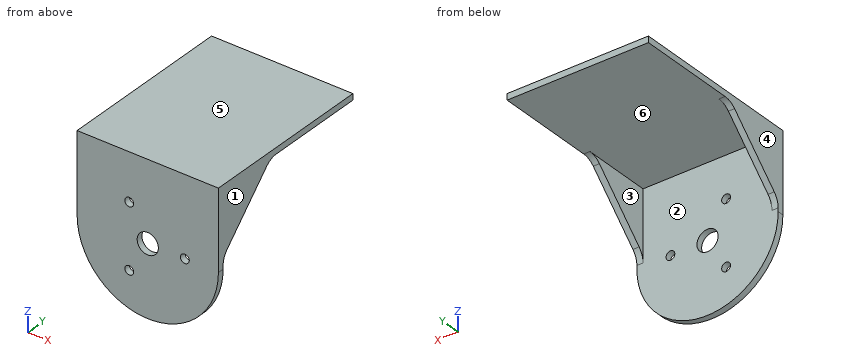
from build123d import *

# Parameters (mm, degrees)
SKETCH1_R            = 2.5
SKETCH1_R_2          = 6
BOSS_EXTRUDE1_DEPTH  = 3.5
SKETCH1_3_W          = 80
SKETCH1_3_H          = 3.5
BOSS_EXTRUDE2_DEPTH  = 100
BOSS_EXTRUDE3_DEPTH  = 3.5
FILLET1_R            = 10
FILLET1_OF_MIRROR1_R = 10


with BuildPart() as part:
    # Sketch1 → Boss-Extrude1 (new body)
    with BuildSketch(Plane(origin=(0, 0, 0), x_dir=(1, 0, 0), z_dir=(0, 1, 0))):
        with BuildLine():
            ThreePointArc((40, 0), (0, 40), (-40, 0))
            Line((-40, 0), (-40, -41.5))
            Line((-40, -41.5), (40, -41.5))
            Line((40, -41.5), (40, 0))
        make_face()
        with Locations((21, 0)):
            Circle(SKETCH1_R, mode=Mode.SUBTRACT)
        with Locations((-10.5, -18.186533479)):
            Circle(SKETCH1_R, mode=Mode.SUBTRACT)
        with Locations((-10.5, 18.186533479)):
            Circle(SKETCH1_R, mode=Mode.SUBTRACT)
        Circle(SKETCH1_R_2, mode=Mode.SUBTRACT)
    extrude(amount=BOSS_EXTRUDE1_DEPTH)

    # Sketch1_3 → Boss-Extrude2 (add)
    with BuildSketch(Plane(origin=(0, 0, 0), x_dir=(1, 0, 0), z_dir=(0, 1, 0))):
        with Locations((0, -43.25)):
            Rectangle(SKETCH1_3_W, SKETCH1_3_H)
    extrude(amount=BOSS_EXTRUDE2_DEPTH)

    # Sketch5 → Boss-Extrude3 (add)
    with BuildSketch(Plane.ZY.offset(40)):
        Polygon((6.144660941, 3.5), (41.5, 38.855339059), (41.5, 3.5), align=None)
    boss_extrude3 = extrude(amount=-BOSS_EXTRUDE3_DEPTH)

    # Fillet1
    fillet1_edges = [part.edges().sort_by_distance(p)[0] for p in [
        (-38.25, 3.5, 6.144660941),
        (-38.25, 38.855339059, 41.5),
    ]]
    fillet(fillet1_edges, radius=FILLET1_R)

    # Mirror1: Boss-Extrude3 across plane
    add(boss_extrude3.mirror(Plane(origin=(0, 0, 0), x_dir=(0, 0, 1), z_dir=(1, 0, 0))))

    # Fillet1 of Mirror1
    fillet1_of_mirror1_edges = [part.edges().sort_by_distance(p)[0] for p in [
        (38.25, 3.5, 6.144660941),
        (38.25, 38.855339059, 41.5),
    ]]
    fillet(fillet1_of_mirror1_edges, radius=FILLET1_OF_MIRROR1_R)


solid = part.part
Build history of the part. All positions in model axes, mm. Face numbers are marked on the shaded views. A direction names the side the tool comes from. Round coordinates to 2 decimals unless told otherwise and drop trailing zeros. Loops run counter-clockwise (first coordinate to the right, second up) from the corner with the lowest first, then second, coordinate; pieces in that order, holes last. Notation, with made-up numbers: (78, 20) -> (116, 20) arc R13 cw to (116, 29) -> close; hole circle Ø9 at (47, 7). An arc over 180 degrees is marked (long way). One line per item, written item: value. Start each with the question number.
Q1. Two-plate mould, pull along X, no slides. Class the marked faces 3, 4, 5 and 6: released by +X, released by -X, zero draft, split by the parting line, or undercut.
Q2. Cut at A-A on x = 0. List the corners of the cut face in (y, z), plus the area to 3 significant figures.
Q3. Probe line 1 along X through (y, z) = (1.5, 0); line 2 along Z through (x, y) = (0, 2); line 3 along Z through (x, y) = (-10.5, 2.55). List the from-to ranges inside material, lowest first.
Q4. Cut at D-D on y = 32. List the corners of the cut face in (x, z).
Q5. Cut at C-C on z = 34.5. List the corners of the cut face in (x, y).
Q6. Drop flat-ended pins along their axis: pin 1 Ø4.5 at (x, z) = (-10.5, 18.19) entering from +Y; pin 2 Ø8 at (x, z) = (-26.5, 7.5) entering from +Y; pin 3 Ø4 at (x, y) = (9.5, 76) entering from -Z. Give the stop position or say it passes through.
Q7. 3-axis set-ups, long thin cutter, end or side, ignore diameter. For the marked faces 1 and 2: which of +Z, -Z, +X, -X, +Y, -Y reach the whole face in a straight line?
Q8. Cut at B-B on x = -10.5. List the corners of the cut face in (y, z), plus the area to 3 significant figures.
Computed:
1. face 3: undercut
1. face 4: released by -X
1. face 5: zero draft
1. face 6: undercut
2. outline: (0, -40) -> (3.5, -40) -> (3.5, -6) -> (0, -6) -> close; (0, 6) -> (3.5, 6) -> (3.5, 41.5) -> (100, 41.5) -> (100, 45) -> (0, 45) -> close
2. area: 593 mm²
3. line 1: -40 to -6, 6 to 18.5, 23.5 to 40
3. line 2: -40 to -6, 6 to 45
3. line 3: -38.6 to -20.69, -15.69 to 15.69, 20.69 to 45
4. outline: (-40, 34.64) -> (-36.5, 34.64) -> (-36.5, 41.5) -> (36.5, 41.5) -> (36.5, 34.64) -> (40, 34.64) -> (40, 45) -> (-40, 45) -> close
5. outline: (-40, 0) -> (40, 0) -> (40, 31.86) -> (36.5, 31.86) -> (36.5, 3.5) -> (-36.5, 3.5) -> (-36.5, 31.86) -> (-40, 31.86) -> close
6. pin 1: through
6. pin 2: y = 3.5
6. pin 3: z = 41.5
7. face 1: +Z, -Z, +X, +Y, -Y
7. face 2: -Z, +Y
8. outline: (0, -38.6) -> (3.5, -38.6) -> (3.5, -20.69) -> (0, -20.69) -> close; (0, -15.69) -> (3.5, -15.69) -> (3.5, 15.69) -> (0, 15.69) -> close; (0, 20.69) -> (3.5, 20.69) -> (3.5, 41.5) -> (100, 41.5) -> (100, 45) -> (0, 45) -> close
8. area: 595 mm²
